Source: CAD feature listing. Evaluate the final solid. Frame: model axes, mm. A direction names the side the tool comes from. Coordinates: 2 decimals unless noted, no trailing zeros. Order: outer loops, then holes, each group sorted by start corner. A loop starts at its lowest first (then second) coordinate and runs counter-clockwise, first axis right, second up. Notation, with made-up numbers: (47, -22.5) - (55, -22.5) arc R27 ccw to (55, -0.5) - close; hole circle Ø2 at (18.25, 89). An arc over 180 degrees is marked (long way). One line per question, with ' | ' between items. Start each with the question number.
(1) Section C-C (y = 0.75). Return the cut outline in (x, z).
(2) Draft query along X for faces 6 (the flat face through (-0.4, 6.985, -30.4)), 7 (the flat face through (22.428, 4.34, -16.509)), 8 (the cylindrical face through (23.825, 0.947, 10.894)). Return one class per face: +X half, -X half, draft (parallel to the pull), parting line (faces both ways), or undercut.
(3) Line query: line 1 along Z through (x, y) = (-19, 2.25); line 2 along Y through (x, z) = (-14, -10.5); line 3 along Z through (x, y) = (1.5, 6.75). Output: solid intervals per line, ascending.
(4) Section A-A (y = 4.5). Return the cut outline in (x, z), then the cut area to 3 significant figures.
(5) Access query for faces 1 (the flat face through (-1, 5, -31.187)), 2 (the flat face through (-24.7, 5.05, -17.13)), 3 (the cylindrical face through (-23.243, 1.596, -16.801)), 4 (the cylindrical face through (-0.8, 0.9, 24.8)), 5 (the flat face through (25.161, 5.053, 7.374)). Directions: +Z, -Z, +X, -X, +Y, -Y. A direction counts if a zero-diameter tool reaches every point of the face in a straight line with its end or side. Return the directions, or none.
(6) Contact query for flat-ended pins moving along their axis: P1, Ø10, axis at x = 8.5, z = -8.5, coming from the +Y side; P2, Ø1, axis at x = 18, y = 5.5, coming from the +Z side; P3, Ø3, axis at x = -4, y = 5, coming from the -Z side. Output: stop coordinate, or through.
from build123d import *

# Parameters (mm, degrees)
BOSS_EXTRUDE1_DEPTH             = 1.5875
BOSS_EXTRUDE2_DEPTH             = 1.5875
FILLET2_R                       = 1.5875
FILLET3_R                       = 3.302
BOSS_EXTRUDE3_DEPTH             = 3.81
BOSS_EXTRUDE3_DIRECTION_2_REACH = 49.633
SKETCH5_R                       = 2.797863207
CUT_EXTRUDE1_DEPTH              = 3.81


# Some blends are built 0.0001 mm under size
with BuildPart() as part:
    # Sketch1 → Boss-Extrude1 (new body)
    with BuildSketch(Plane(origin=(0, 0, 0), x_dir=(1, 0, 0), z_dir=(0, 1, 0))):
        Polygon((-34.41906837, 3.470841979), (-17.500524818, -25.832935043), (16.336562287, -25.832935043), (33.255105839, 3.470841979), (16.336562287, 32.774619002), (-17.500524818, 32.774619002), align=None)
    extrude(amount=BOSS_EXTRUDE1_DEPTH)

    # Sketch2 → Boss-Extrude2 (add)
    # profile 1 of 3: a face of its own
    with BuildSketch(Plane(origin=(0, 1.5875, 0), x_dir=(1, 0, 0), z_dir=(0, 1, 0))):
        Polygon((16.336562287, 32.774619002), (-17.500524818, 32.774619002), (-34.41906837, 3.470841979), (-17.500524818, -25.832935043), (16.336562287, -25.832935043), (33.255105839, 3.470841979), align=None)
        Polygon((-32.585981265, 3.470841979), (-16.583981265, 31.187119002), (15.420018735, 31.187119002), (31.422018735, 3.470841979), (15.420018735, -24.245435043), (-16.583981265, -24.245435043), align=None, mode=Mode.SUBTRACT)
    # profile 2 of 3: a face of its own
    with BuildSketch(Plane(origin=(0, 1.5875, 0), x_dir=(1, 0, 0), z_dir=(0, 1, 0))):
        Polygon((16.336562287, 32.774619002), (-17.500524818, 32.774619002), (-34.41906837, 3.470841979), (-17.500524818, -25.832935043), (16.336562287, -25.832935043), (33.255105839, 3.470841979), align=None)
        Polygon((-32.585981265, 3.470841979), (-16.583981265, 31.187119002), (15.420018735, 31.187119002), (31.422018735, 3.470841979), (15.420018735, -24.245435043), (-16.583981265, -24.245435043), align=None, mode=Mode.SUBTRACT)
    # profile 3 of 3: a face of its own
    with BuildSketch(Plane(origin=(0, 1.5875, 0), x_dir=(1, 0, 0), z_dir=(0, 1, 0))):
        Polygon((33.255105839, 3.470841979), (16.336562287, 32.774619002), (-17.500524818, 32.774619002), (-34.41906837, 3.470841979), (-17.500524818, -25.832935043), (16.336562287, -25.832935043), align=None)
        Polygon((-16.583981265, -24.245435043), (-32.585981265, 3.470841979), (-16.583981265, 31.187119002), (15.420018735, 31.187119002), (31.422018735, 3.470841979), (15.420018735, -24.245435043), align=None, mode=Mode.SUBTRACT)
    extrude(amount=BOSS_EXTRUDE2_DEPTH)

    # Fillet2
    fillet2_edges = [part.edges().sort_by_distance(p)[0] for p in [
        (23.421018735, 1.5875, -17.328980491),
        (23.421018735, 1.5875, 10.387296532),
        (-24.584981265, 1.5875, -17.328980491),
        (-0.581981265, 1.5875, 24.245435043),
        (-24.584981265, 1.5875, 10.387296532),
        (-0.581981265, 1.5875, -31.187119002),
    ]]
    fillet(fillet2_edges, radius=FILLET2_R - 0.0001)  # a hair under: the kernel refuses the full size

    # Fillet3
    # the kernel refuses this fillet: 3.302 mm, written as the material it takes off along each edge
    with BuildSketch(Plane(origin=(-25.749416789, 0, 25.832935043), x_dir=(0, 1, 0), z_dir=(1, 0, 0)), Plane(origin=(-38.543514355, 0, -10.614591979), x_dir=(0, 1, 0), z_dir=(0.4999999999999999, 0, 0.8660254037844387)), Plane(origin=(-13.376078832, 0, -39.918369002), x_dir=(0, 1, 0), z_dir=(-0.5000000000000002, 0, 0.8660254037844386)), Plane(origin=(24.585454258, 0, -32.774619002), x_dir=(0, 1, 0), z_dir=(-1, 0, 0)), Plane(origin=(12.212116302, 0, 32.976685043), x_dir=(0, 1, 0), z_dir=(0.5000000000000001, 0, -0.8660254037844387)), Plane(origin=(37.379551825, 0, 3.672908021), x_dir=(0, 1, 0), z_dir=(-0.5, 0, -0.8660254037844387))) as fillet3_piece_1:
        with BuildLine():
            CenterArc((3.302, -3.299556788), FILLET3_R, 92.204227504, 87.795772496)
            Line((0, -3.299556788), (-0.06604, -3.299556788))
            Line((-0.06604, -3.299556788), (-0.06604, 0))
            Line((-0.06604, 0), (0, 0.06604))
            ThreePointArc((0, 0.06604), (1.5875, 0.06604), (3.17246, 0.065991136))
            Line((3.17246, 0.065991136), (3.175, 0))
        make_face()
    extrude(amount=50.334871047, mode=Mode.SUBTRACT)

    # Sketch4 → Boss-Extrude3 (add)
    with BuildSketch(Plane(origin=(0, 3.175, 0), x_dir=(1, 0, 0), z_dir=(0, 1, 0))):
        Polygon((-32.585981265, 3.470841979), (-16.583981265, 31.187119002), (15.420018735, 31.187119002), (31.422018735, 3.470841979), (18.722018735, -18.526203277), (17.622166472, -17.891203277), (29.955549051, 3.470841979), (14.686783893, 29.917119002), (-15.850746423, 29.917119002), (-31.119511582, 3.470841979), (-18.786129002, -17.891203277), (-19.885981265, -18.526203277), align=None)
    extrude(amount=BOSS_EXTRUDE3_DEPTH)

    # Sketch4 → Boss-Extrude3 direction 2 (add, up to next)
    with BuildSketch(Plane(origin=(0, 3.175, 0), x_dir=(1, 0, 0), z_dir=(0, 1, 0)), mode=Mode.PRIVATE) as boss_extrude3_direction_2_sk1:
        Polygon((-32.585981265, 3.470841979), (-16.583981265, 31.187119002), (15.420018735, 31.187119002), (31.422018735, 3.470841979), (18.722018735, -18.526203277), (17.622166472, -17.891203277), (29.955549051, 3.470841979), (14.686783893, 29.917119002), (-15.850746423, 29.917119002), (-31.119511582, 3.470841979), (-18.786129002, -17.891203277), (-19.885981265, -18.526203277), align=None)
    boss_extrude3_direction_2_tool1 = extrude(boss_extrude3_direction_2_sk1.sketch, amount=-BOSS_EXTRUDE3_DIRECTION_2_REACH, mode=Mode.PRIVATE) - part.part
    add(boss_extrude3_direction_2_tool1.solids().sort_by_distance((-23.883103, 3.175, -16.923751))[0])

    # Sketch5 → Cut-Extrude1 (cut)
    with BuildSketch(Plane(origin=(0, 1.5875, 0), x_dir=(1, 0, 0), z_dir=(0, 1, 0))):
        with Locations(Location((17.401743672, -1.065074689, 0), (0, 0, 270))):
            Circle(SKETCH5_R)
    extrude(amount=-CUT_EXTRUDE1_DEPTH, mode=Mode.SUBTRACT)


solid = part.part
Response values:
1) outline: (-33.03, -3.47) - (-16.81, -31.57) - (15.64, -31.57) - (31.86, -3.47) - (15.64, 24.63) - (-16.81, 24.63) - close; hole circle Ø5.6 at (17.4, 1.07)
2) face 6: draft | face 7: undercut | face 8: +X half
3) line 1: z = -29.84 to -24.46, 17.52 to 18.01, 19.47 to 22.9 | line 2: y = 0 to 1.59 | line 3: z = -31.19 to -29.92
4) outline: (-32.59, -3.47) - (-16.58, -31.19) - (15.42, -31.19) - (31.42, -3.47) - (18.72, 18.53) - (17.62, 17.89) - (29.96, -3.47) - (14.69, -29.92) - (-15.85, -29.92) - (-31.12, -3.47) - (-18.79, 17.89) - (-19.89, 18.53) - close | area: 183 mm²
5) face 1: -Z, +X, -X, +Y | face 2: -Z, -X, +Y | face 3: +Y | face 4: +Z, +X, -X, -Y | face 5: +Z, +X, +Y
6) P1: stops at y = 1.59 | P2: stops at z = 18.4 | P3: stops at z = -31.19
